```python
from build123d import *

# Parameters (mm, degrees)
F1_DEPTH = 6.604


with BuildPart() as f1:
    # F0 (on Top) → F1 (new body)
    with BuildSketch(Plane.XY):
        Polygon((-88.9, 88.9), (0, 0), (88.9, 88.9), (0, 88.9), align=None)
        with BuildLine():
            ThreePointArc((0, 23.6728), (-32.5308292905, 56.2864), (0, 88.9))
            ThreePointArc((0, 88.9), (22.0701917215, 80.3739843781), (32.5687625572, 59.1710054502))
            ThreePointArc((32.5687625572, 59.1710054502), (32.6646109516, 57.7301179639), (32.6965813095, 56.2864))
            ThreePointArc((32.6965813095, 56.2864), (23.1149284543, 33.1957453196), (0, 23.6728))
        make_face(mode=Mode.SUBTRACT)
        with BuildLine():
            Line((88.9, 88.9), (0, 0))
            Line((0, 0), (88.9, -88.9))
            Line((88.9, -88.9), (88.9, -1.303055018))
            ThreePointArc((88.9, -1.303055018), (78.2779390849, -24.7410549975), (53.9692081511, -33.1822410226))
            ThreePointArc((53.9692081511, -33.1822410226), (32.2033809996, -22.6365581058), (23.6858169762, 0))
            ThreePointArc((23.6858169762, 0), (56.2929084881, 31.962072491), (88.9, 0))
            Line((88.9, 0), (88.9, 88.9))
        make_face()
        with BuildLine():
            Line((-88.9, -88.9), (0, -88.9))
            ThreePointArc((0, -88.9), (-23.4333822085, -78.7489741197), (-32.3691311793, -54.8257820567))
            ThreePointArc((-32.3691311793, -54.8257820567), (-22.4036802199, -32.787394799), (0, -23.6728))
            ThreePointArc((0, -23.6728), (23.1989938683, -33.1496268937), (32.826729568, -56.2864))
            ThreePointArc((32.826729568, -56.2864), (23.3492107959, -79.2729561788), (0.4248753792, -88.9))
            Line((0.4248753792, -88.9), (88.9, -88.9))
            Line((88.9, -88.9), (0, 0))
            Line((0, 0), (-88.9, -88.9))
        make_face()
        with BuildLine():
            Line((-88.9, 0), (-88.9, -88.9))
            Line((-88.9, -88.9), (0, 0))
            Line((0, 0), (-88.9, 88.9))
            Line((-88.9, 88.9), (-88.9, 3.0109182433))
            ThreePointArc((-88.9, 3.0109182433), (-79.5055607914, 24.4438044642), (-58.1749416888, 34.0681895614))
            ThreePointArc((-58.1749416888, 34.0681895614), (-33.9222205657, 25.2151766333), (-23.7036289165, 1.5054591217))
            ThreePointArc((-23.7036289165, 1.5054591217), (-23.7123207699, 0.7525289094), (-23.7383916974, 0))
            ThreePointArc((-23.7383916974, 0), (-56.3191958487, -31.1101078106), (-88.9, 0))
        make_face()
        with BuildLine():
            Line((0, 23.6728), (0, 88.9))
            ThreePointArc((0, 88.9), (-32.5308292905, 56.2864), (0, 23.6728))
        make_face()
        with BuildLine():
            Line((56.2929084881, -0.651527509), (88.9, 0))
            ThreePointArc((88.9, 0), (56.2929084881, 31.962072491), (23.6858169762, 0))
            Line((23.6858169762, 0), (56.2929084881, -0.651527509))
        make_face()
        with BuildLine():
            Line((-23.7383916974, 0), (-88.9, 0))
            ThreePointArc((-88.9, 0), (-56.3191958487, -31.1101078106), (-23.7383916974, 0))
        make_face()
        with BuildLine():
            Line((-58.1749416888, 34.0681895614), (-23.7383916974, 0))
            ThreePointArc((-23.7383916974, 0), (-23.7123207699, 0.7525289094), (-23.7036289165, 1.5054591217))
            ThreePointArc((-23.7036289165, 1.5054591217), (-33.9222205657, 25.2151766333), (-58.1749416888, 34.0681895614))
        make_face()
        with BuildLine():
            ThreePointArc((-32.3691311793, -54.8257820567), (-23.4333822085, -78.7489741197), (0, -88.9))
            Line((0, -88.9), (-32.3691311793, -54.8257820567))
        make_face()
        with BuildLine():
            ThreePointArc((0, -23.6728), (-22.4036802199, -32.787394799), (-32.3691311793, -54.8257820567))
            Line((-32.3691311793, -54.8257820567), (0, -23.6728))
        make_face()
    extrude(amount=-F1_DEPTH)


solid = f1.part
```
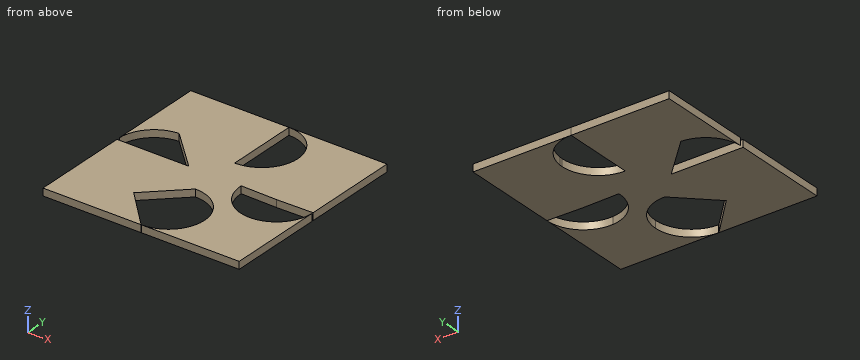
Part model, mm, in its own coordinate system. Coordinates: 2 decimals unless noted, no trailing zeros. Write each loop counter-clockwise with the first axis right and the second up, starting at its lowest first coordinate (ties: lowest second). Pieces come first, ordered by that corner, then holes.
Item 1: Slice it at B-B (x = -13.5). Write the cut outline in (y, z).
Item 2: Probe line 1 (Y direction, x = 58.5, z = -5.75); line 2 (X direction, y = 55, z = -3.5); line 3 (Y direction, x = 21.5, z = -3.5). List the from-to ranges inside material, lowest first.
Item 3: Slice it at A-A (y = 75.5). Write the cut outline in (x, z).
Item 4: Slice it at D-D (x = 11). Write the cut outline in (y, z), and give its area (3 significant figures).
Item 5: Slice it at C-C (z = -5.25). Write the cut outline in (x, y).
Results found:
1. outline: (-88.9, -6.6) - (-74.69, -6.6) - (-74.69, 0) - (-88.9, 0) - close; (-36.67, -6.6) - (88.9, -6.6) - (88.9, 0) - (-36.67, 0) - close
2. line 1: y = -88.9 to -33.19, -0.61 to 88.9
2. line 2: x = -88.9 to 0, 32.67 to 88.9
2. line 3: y = -88.9 to -81, -31.58 to 31.69, 80.88 to 88.9
3. outline: (-88.9, -6.6) - (0, -6.6) - (0, 0) - (-88.9, 0) - close; (26.44, -6.6) - (88.9, -6.6) - (88.9, 0) - (26.44, 0) - close
4. outline: (-88.9, -6.6) - (-87.06, -6.6) - (-87.06, 0) - (-88.9, 0) - close; (-25.51, -6.6) - (25.55, -6.6) - (25.55, 0) - (-25.51, 0) - close; (87.02, -6.6) - (88.9, -6.6) - (88.9, 0) - (87.02, 0) - close
4. area: 362 mm2
5. outline: (-88.9, -88.9) - (0, -88.9) - (-32.37, -54.83) - (0, -23.67) arc R32.61 cw to (0.42, -88.9) - (88.9, -88.9) - (88.9, -1.3) arc R32.61 cw to (23.69, 0) - (56.29, -0.65) - (88.9, 0) - (88.9, 88.9) - (0.17, 88.9) arc R32.61 cw to (0, 23.67) - (0, 88.9) - (-88.9, 88.9) - (-88.9, 3.01) arc R32.62 cw to (-58.17, 34.07) - (-23.74, 0) - (-88.9, 0) - close
